Part print with two shaded views. Sizes in mm from the minimum x, y, z corner. A direction names the side the tool comes from. Round coordinates to 2 decimals unless told otherwise and drop trailing zeros. Order: outer loops, then holes, each group sorted by start corner. A loop starts at its lowest first (then second) coordinate and runs counter-clockwise, first axis right, second up. Notation, with made-up numbers: (50.25, 18.5) -> (69.25, 18.5) arc R24 ccw to (69.25, 29.5) -> close; hole circle Ø4 at (49, 31.5). An arc over 180 degrees is marked (long way). Put each result on its own line as item: value. Start each with the question number.
Q1. Cut at B-B, the plane x = 11. List the corners of the cut face in (y, z).
Q2. Cut at C-C, the plane z = 49.5. List the corners of the cut face in (x, y), and give its area (3 significant figures).
Q3. Flat gauge pins, fed straight in: P1, Ø6.5, axis at x = 23.5, y = 10, coming from the -Z side; P2, Ø3, axis at x = 47.5, z = 46, coming from the +Y side. Where does each tip first touch, or does it go through?
Q4. Probe L1, parallel to X at y = 15.25, z = 46; L2, parallel to Y at x = 44, z = 43. List the from-to ranges inside material, lowest first.
Q5. Pull direction X, two halves, no side cores. Call the marked faces 1, 2 and 3: released by +X, released by -X, zero draft, split by the parting line, or undercut.
Q6. 3-axis set-ups, long thin cutter, end or side, ignore diameter. For the marked faces 4 and 5: which of +Z, -Z, +X, -X, +Y, -Y reach the whole face in a straight line?
Q7. Cut at A-A, the plane y = 14.25. List the corners of the cut face in (x, z), and give its area (3 significant figures).
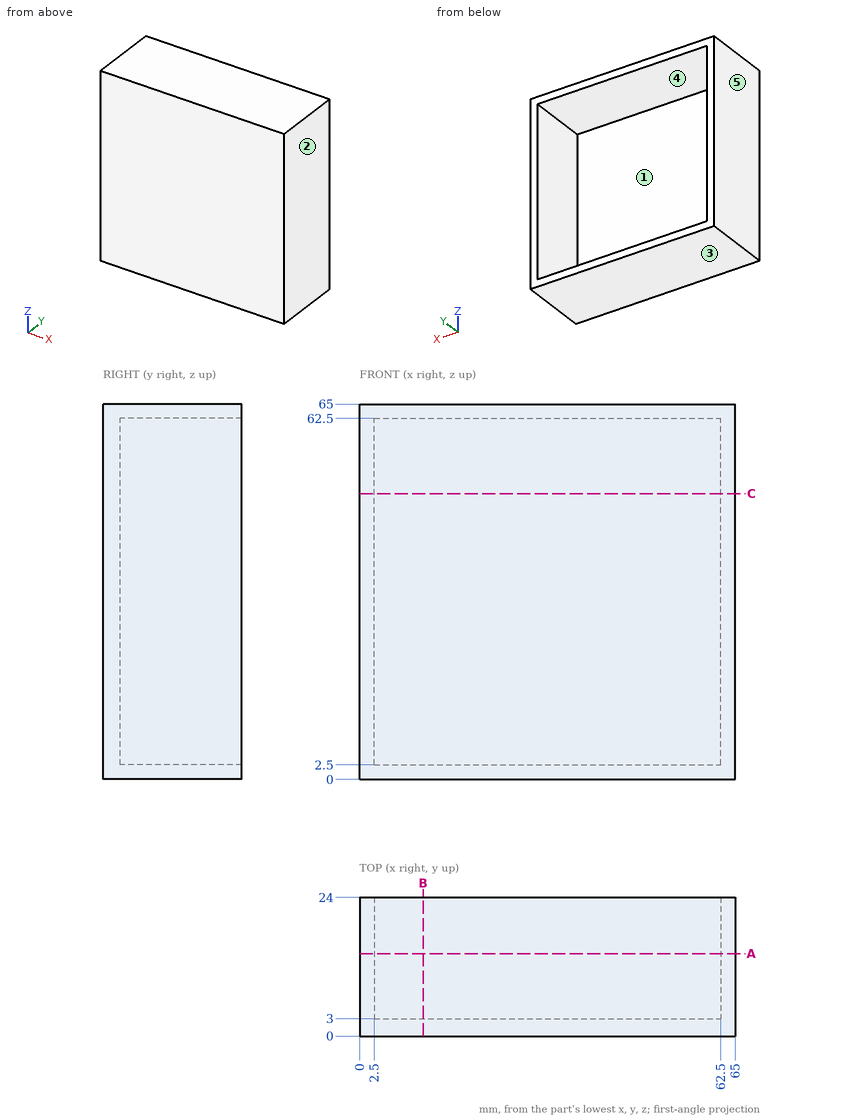
Ans:
1. outline: (0, 0) -> (24, 0) -> (24, 2.5) -> (3, 2.5) -> (3, 62.5) -> (24, 62.5) -> (24, 65) -> (0, 65) -> close
2. outline: (0, 0) -> (65, 0) -> (65, 24) -> (62.5, 24) -> (62.5, 3) -> (2.5, 3) -> (2.5, 24) -> (0, 24) -> close
2. area: 300 mm^2
3. P1: stops at z = 0
3. P2: stops at y = 3
4. L1: x = 0 to 2.5, 62.5 to 65
4. L2: y = 0 to 3
5. face 1: undercut
5. face 2: released by +X
5. face 3: zero draft
6. face 4: +Y
6. face 5: +Z, -Z, -X, +Y, -Y
7. outline: (0, 0) -> (65, 0) -> (65, 65) -> (0, 65) -> close; hole (2.5, 2.5) -> (62.5, 2.5) -> (62.5, 62.5) -> (2.5, 62.5) -> close
7. area: 625 mm^2
